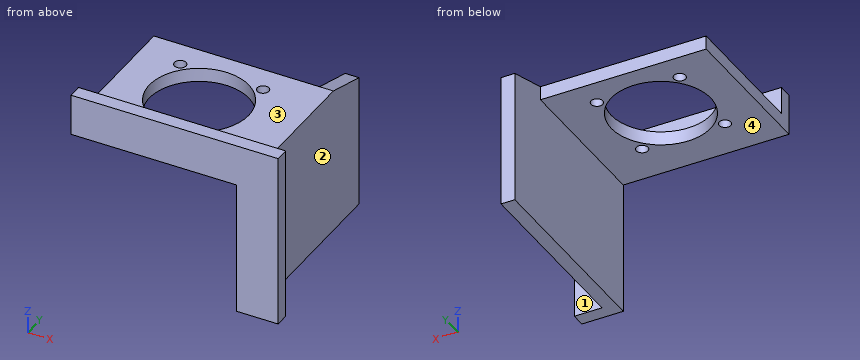
```python
from build123d import *

# Parameters (mm, degrees)
SKETCH1_W           = 120
SKETCH1_H           = 110
SKETCH1_R           = 4.25
SKETCH1_R_2         = 36
BOSS_EXTRUDE1_DEPTH = 10
SKETCH2_W           = 107
SKETCH2_H           = 144
BOSS_EXTRUDE2_DEPTH = 10
CHAMFER1_SIZE       = 10
CHAMFER1_SIZE2      = 34
BOSS_EXTRUDE4_DEPTH = 10


with BuildPart() as part:
    # Sketch1 → Boss-Extrude1 (new body)
    with BuildSketch(Plane.XY):
        with Locations((-30, -35)):
            Rectangle(SKETCH1_W, SKETCH1_H)
        Circle(SKETCH1_R, mode=Mode.SUBTRACT)
        with Locations((0, -60)):
            Circle(SKETCH1_R, mode=Mode.SUBTRACT)
        with Locations((-30, -30)):
            Circle(SKETCH1_R_2, mode=Mode.SUBTRACT)
        with Locations(Location((-60, 0, 0), (0, 0, 180))):
            Circle(SKETCH1_R, mode=Mode.SUBTRACT)
        with Locations(Location((-60, -60, 0), (0, 0, 180))):
            Circle(SKETCH1_R, mode=Mode.SUBTRACT)
    extrude(amount=BOSS_EXTRUDE1_DEPTH)

    # Sketch2 → Boss-Extrude2 (add)
    with BuildSketch(Plane(origin=(30, 0, 0), x_dir=(0, 0, -1), z_dir=(1, 0, 0))):
        with Locations((43.5, -18)):
            Rectangle(SKETCH2_W, SKETCH2_H)
    extrude(amount=BOSS_EXTRUDE2_DEPTH)

    # Chamfer1
    chamfer1_edges = [part.edges().sort_by_distance(p)[0] for p in [
        (35, 54, 10),
    ]]
    chamfer1_side = [part.faces().sort_by_distance(p)[0] for p in [
        (35, 54, -43.5),
    ]]
    chamfer(chamfer1_edges, length=CHAMFER1_SIZE, length2=CHAMFER1_SIZE2, reference=chamfer1_side[0])

    # Sketch6 → Boss-Extrude4 (add)
    with BuildSketch(Plane.XZ.offset(90)):
        Polygon((-90, 30), (-90, 10), (40, 10), (40, -97), (60, -97), (60, 30), align=None)
    extrude(amount=-BOSS_EXTRUDE4_DEPTH)


solid = part.part
```
Read the model definition and answer for the solid it produces. Units are mm, in the model's axes. Face numbers are marked on the shaded views. A direction names the side the tool comes from. Coordinates: 2 decimals unless noted, no trailing zeros. Loops run counter-clockwise (first coordinate to the right, second up) from the corner with the lowest first, then second, coordinate; pieces in that order, holes last. Notation, with made-up numbers: (39, 12) - (61, 12) arc R21 ccw to (61, 18) - close; hole circle Ø5 at (68.5, 1.5). An arc over 180 degrees is marked (long way). Answer in a Markdown table with one row per item.
1. Find section D-D, the plane y = -60. Write down the section's boundary in (x, z).
Conclusion:
| item | result |
|---|---|
| outline | (-90, 0) - (-64.25, 0) - (-64.25, 10) - (-90, 10) - close; (-55.75, 0) - (-49.9, 0) - (-49.9, 10) - (-55.75, 10) - close; (-10.1, 0) - (-4.25, 0) - (-4.25, 10) - (-10.1, 10) - close; (4.25, 0) - (30, 0) - (30, -97) - (40, -97) - (40, 10) - (4.25, 10) - close |
2. Given pin 1 (10 mm diameter, centred on x = 38.5, y = 9.5, fed in from +Z); pin 2 (13.5 mm diameter, centred on x = -60, y = -60, fed in from -Z); pin 3 (12 mm diameter, centred on y = -49, z = -74.5, fed in from +X), each flat-ended and moving along its own axis, determine where each tip first touches the part or whether it passes through.
Conclusion:
| item | result |
|---|---|
| pin 1 | stops at z = 10 |
| pin 2 | stops at z = 0 |
| pin 3 | stops at x = 40 |
3. Find section C-C, the plane z = -64.5. Write down the section's boundary in (x, y).
Conclusion:
| item | result |
|---|---|
| outline | (30, -90) - (60, -90) - (60, -80) - (40, -80) - (40, 54) - (30, 54) - close |
4. Find section A-A, the plane y = -30. Write down the section's boundary in (x, z), then the cut area to 3 significant figures.
Conclusion:
| item | result |
|---|---|
| outline | (-90, 0) - (-66, 0) - (-66, 10) - (-90, 10) - close; (6, 0) - (30, 0) - (30, -97) - (40, -97) - (40, 10) - (6, 10) - close |
| area | 1,550 mm² |
5. Find section B-B, the plane x = -30. Write down the section's boundary in (y, z), then the cut area to 3 significant figures.
Conclusion:
| item | result |
|---|---|
| outline | (-90, 0) - (-66, 0) - (-66, 10) - (-80, 10) - (-80, 30) - (-90, 30) - close; (6, 0) - (20, 0) - (20, 10) - (6, 10) - close |
| area | 580 mm² |
6. Which of the six approach directions +Z, -Z, +X, -X, +Y, -Y give full straight-line access (tool end or side, diameter ignored) to the marked faces 1, 2, 3 and 4?
Conclusion:
| item | result |
|---|---|
| face 1 | +Z, +X, +Y |
| face 2 | +Z, -Z, +X, +Y |
| face 3 | +Z, +X, -X, +Y |
| face 4 | -Z, -X, +Y, -Y |
7. Straight lines are drawn through the part: line 1 (Y direction, x = -60, z = 4); line 2 (X direction, y = 18, z = -31.5); line 3 (Y direction, x = -36, z = 12.5). For each, find the intervals that lie inside material, in ascending order.
Conclusion:
| item | result |
|---|---|
| line 1 | y = -90 to -64.25, -55.75 to -49.9, -10.1 to -4.25, 4.25 to 20 |
| line 2 | x = 30 to 40 |
| line 3 | y = -90 to -80 |
